```python
from build123d import *

# Parameters (mm, degrees)
SKETCH_1_W          = 44
SKETCH_1_H          = 30
EXTRUDE_1_DEPTH     = 24
SKETCH_5_W          = 20
SKETCH_5_H          = 34.070761632
CUT_EXTRUDE_3_DEPTH = 20
SKETCH_6_R          = 1.5
CUT_EXTRUDE_4_DEPTH = 44
FILLET_1_R          = 2
FILLET_2_R          = 2


# Some blends are built 0.0001 mm under size
with BuildPart() as part:
    # 草图1 → 凸台-拉伸1 (new body)
    with BuildSketch(Plane.XY):
        Rectangle(SKETCH_1_W, SKETCH_1_H)
    extrude(amount=EXTRUDE_1_DEPTH)

    # 草图5 → 切除-拉伸3 (cut)
    with BuildSketch(Plane.XY.offset(24)):
        with Locations((0, 0.619885825)):
            Rectangle(SKETCH_5_W, SKETCH_5_H)
    extrude(amount=-CUT_EXTRUDE_3_DEPTH, mode=Mode.SUBTRACT)

    # 草图6 → 切除-拉伸4 (cut)
    with BuildSketch(Plane(origin=(22, 0, 0), x_dir=(0, 0, -1), z_dir=(1, 0, 0))):
        with Locations((-19, 5)):
            Circle(SKETCH_6_R)
        with Locations((-19, -5)):
            Circle(SKETCH_6_R)
        with Locations((-9, -5)):
            Circle(SKETCH_6_R)
        with Locations((-9, 5)):
            Circle(SKETCH_6_R)
    extrude(amount=-CUT_EXTRUDE_4_DEPTH, mode=Mode.SUBTRACT)

    # 圆角1
    fillet_1_edges = [part.edges().sort_by_distance(p)[0] for p in [
        (-16, -15, 24),
        (-16, 15, 24),
        (16, -15, 24),
        (0, -15, 4),
        (0, 15, 4),
        (-10, 15, 14),
        (-10, -15, 14),
        (10, 15, 14),
        (10, -15, 14),
        (0, -15, 0),
        (0, 15, 0),
        (16, 15, 24),
        (22, -15, 12),
        (-22, -15, 12),
        (-22, 15, 12),
        (22, 15, 12),
    ]]
    fillet(fillet_1_edges, radius=FILLET_1_R - 0.0001)  # a hair under: the kernel refuses the full size

    # 圆角2
    # the kernel refuses this fillet: 2 mm, written as the material it takes off along each edge
    with BuildSketch(Plane(origin=(-12, -15, 22), x_dir=(1, 0, 0), z_dir=(0, 0, -1))) as fillet_2_piece_1:
        with BuildLine():
            CenterArc((0.0001, -1.9999), 1.9999, 0, 90)
            Line((2, -1.9999), (2, 0))
            Line((2, 0), (0.0001, 0))
        make_face()
    revolve(axis=Axis((-12, -15, 22), (0, -1, 0)), revolution_arc=90, mode=Mode.SUBTRACT)
    with BuildSketch(Plane(origin=(-20, -15, 22), x_dir=(0, 0, 1), z_dir=(1, 0, 0))) as fillet_2_piece_2:
        with BuildLine():
            CenterArc((0.0001, -1.9999), 1.9999, 0, 90)
            Line((2, -1.9999), (2, 0))
            Line((2, 0), (0.0001, 0))
        make_face()
    revolve(axis=Axis((-20, -15, 22), (0, -1, 0)), revolution_arc=90, mode=Mode.SUBTRACT)
    with BuildSketch(Plane(origin=(-20, -15, 2), x_dir=(-1, 0, 0), z_dir=(0, 0, 1))) as fillet_2_piece_3:
        with BuildLine():
            CenterArc((0.0001, -1.9999), 1.9999, 0, 90)
            Line((2, -1.9999), (2, 0))
            Line((2, 0), (0.0001, 0))
        make_face()
    revolve(axis=Axis((-20, -15, 2), (0, -1, 0)), revolution_arc=90, mode=Mode.SUBTRACT)
    with BuildSketch(Plane(origin=(20, -15, 2), x_dir=(0, 0, -1), z_dir=(-1, 0, 0))) as fillet_2_piece_4:
        with BuildLine():
            CenterArc((0.0001, -1.9999), 1.9999, 0, 90)
            Line((2, -1.9999), (2, 0))
            Line((2, 0), (0.0001, 0))
        make_face()
    revolve(axis=Axis((20, -15, 2), (0, -1, 0)), revolution_arc=90, mode=Mode.SUBTRACT)
    with BuildSketch(Plane(origin=(12, -15, 22), x_dir=(0, 0, 1), z_dir=(1, 0, 0))) as fillet_2_piece_5:
        with BuildLine():
            CenterArc((0.0001, -1.9999), 1.9999, 0, 90)
            Line((2, -1.9999), (2, 0))
            Line((2, 0), (0.0001, 0))
        make_face()
    revolve(axis=Axis((12, -15, 22), (0, -1, 0)), revolution_arc=90, mode=Mode.SUBTRACT)
    with BuildSketch(Plane(origin=(20, -15, 22), x_dir=(1, 0, 0), z_dir=(0, 0, -1))) as fillet_2_piece_6:
        with BuildLine():
            CenterArc((0.0001, -1.9999), 1.9999, 0, 90)
            Line((2, -1.9999), (2, 0))
            Line((2, 0), (0.0001, 0))
        make_face()
    revolve(axis=Axis((20, -15, 22), (0, -1, 0)), revolution_arc=90, mode=Mode.SUBTRACT)
    with BuildSketch(Plane(origin=(12, 15, 22), x_dir=(-1, 0, 0), z_dir=(0, 0, -1))) as fillet_2_piece_7:
        with BuildLine():
            CenterArc((0.0001, -1.9999), 1.9999, 0, 90)
            Line((2, -1.9999), (2, 0))
            Line((2, 0), (0.0001, 0))
        make_face()
    revolve(axis=Axis((12, 15, 22), (0, 1, 0)), revolution_arc=90, mode=Mode.SUBTRACT)
    with BuildSketch(Plane(origin=(20, 15, 22), x_dir=(0, 0, 1), z_dir=(-1, 0, 0))) as fillet_2_piece_8:
        with BuildLine():
            CenterArc((0.0001, -1.9999), 1.9999, 0, 90)
            Line((2, -1.9999), (2, 0))
            Line((2, 0), (0.0001, 0))
        make_face()
    revolve(axis=Axis((20, 15, 22), (0, 1, 0)), revolution_arc=90, mode=Mode.SUBTRACT)
    with BuildSketch(Plane(origin=(-12, 15, 22), x_dir=(0, 0, 1), z_dir=(-1, 0, 0))) as fillet_2_piece_9:
        with BuildLine():
            CenterArc((0.0001, -1.9999), 1.9999, 0, 90)
            Line((2, -1.9999), (2, 0))
            Line((2, 0), (0.0001, 0))
        make_face()
    revolve(axis=Axis((-12, 15, 22), (0, 1, 0)), revolution_arc=90, mode=Mode.SUBTRACT)
    with BuildSketch(Plane(origin=(20, 15, 2), x_dir=(1, 0, 0), z_dir=(0, 0, 1))) as fillet_2_piece_10:
        with BuildLine():
            CenterArc((0.0001, -1.9999), 1.9999, 0, 90)
            Line((2, -1.9999), (2, 0))
            Line((2, 0), (0.0001, 0))
        make_face()
    revolve(axis=Axis((20, 15, 2), (0, 1, 0)), revolution_arc=90, mode=Mode.SUBTRACT)
    with BuildSketch(Plane(origin=(-20, 15, 22), x_dir=(-1, 0, 0), z_dir=(0, 0, -1))) as fillet_2_piece_11:
        with BuildLine():
            CenterArc((0.0001, -1.9999), 1.9999, 0, 90)
            Line((2, -1.9999), (2, 0))
            Line((2, 0), (0.0001, 0))
        make_face()
    revolve(axis=Axis((-20, 15, 22), (0, 1, 0)), revolution_arc=90, mode=Mode.SUBTRACT)
    with BuildSketch(Plane(origin=(-20, 15, 2), x_dir=(0, 0, -1), z_dir=(1, 0, 0))) as fillet_2_piece_12:
        with BuildLine():
            CenterArc((0.0001, -1.9999), 1.9999, 0, 90)
            Line((2, -1.9999), (2, 0))
            Line((2, 0), (0.0001, 0))
        make_face()
    revolve(axis=Axis((-20, 15, 2), (0, 1, 0)), revolution_arc=90, mode=Mode.SUBTRACT)
    with BuildSketch(Plane(origin=(-22, 15, 0), x_dir=(0, 0, 1), z_dir=(0, -1, 0)), Plane(origin=(-22, 15, 24), x_dir=(1, 0, 0), z_dir=(0, -1, 0)), Plane(origin=(10, -15, 24), x_dir=(0, 0, -1), z_dir=(0, 1, 0))) as fillet_2_piece_13:
        with BuildLine():
            CenterArc((FILLET_2_R, -FILLET_2_R), FILLET_2_R, 90, 90)
            Line((0, -FILLET_2_R), (0, 0))
            Line((0, 0), (FILLET_2_R, 0))
        make_face()
    extrude(amount=30, mode=Mode.SUBTRACT)
    with BuildSketch(Plane(origin=(22, -15, 0), x_dir=(-1, 0, 0), z_dir=(0, 1, 0)), Plane(origin=(22, -15, 24), x_dir=(0, 0, -1), z_dir=(0, 1, 0)), Plane(origin=(-10, 15, 24), x_dir=(-1, 0, 0), z_dir=(0, -1, 0))) as fillet_2_piece_14:
        with BuildLine():
            CenterArc((FILLET_2_R, FILLET_2_R), FILLET_2_R, 180, 90)
            Line((0, FILLET_2_R), (0, 0))
            Line((0, 0), (FILLET_2_R, 0))
        make_face()
    extrude(amount=30, mode=Mode.SUBTRACT)


solid = part.part
```
Can you work these out from the model? Positions are in its coordinate system, mm. A direction names the side the tool comes from. Give positions to 0.01 mm unless a question says otherwise; leave off trailing zeros. Order: outer loops, then holes, each group sorted by start corner. A loop starts at its lowest first (then second) coordinate and runs counter-clockwise, first axis right, second up. Notation, with made-up numbers: M 29,9 L 70,9 A22 ccw 70,47 Z; hole C 57.25,89.5 d8. An arc over 180 degrees is marked long. One line per item, written item: value.
1) On a 3-axis mill with a long thin cutter (end or side, diameter ignored), from which of +Z, -Z, +X, -X, +Y, -Y can I reach the whole of each face in a straight line? I mean faces 5 (the face through (-10.6, -14.43, 11.86)), 6 (the face through (21.4, -0.18, 23.43)), 7 (the face through (0, 0, 4)). Say none if no direction works.
Answer sheet:
face 5: +Z, -Y
face 6: +Z, +X, +Y, -Y
face 7: +Z, +Y, -Y
2) I want a section at D-D, the plane z = 12.75. List the corners of the cut face in (x, y) for me, plus the area to 3 significant figures.
Answer sheet:
outline: M -22,-13 A2 ccw -20,-15 L -12,-15 A2 ccw -10,-13 L -10,13 A2 ccw -12,15 L -20,15 A2 ccw -22,13 Z; M 10,-13 A2 ccw 12,-15 L 20,-15 A2 ccw 22,-13 L 22,13 A2 ccw 20,15 L 12,15 A2 ccw 10,13 Z
area: 713 mm^2
3) I want a section at B-B, the plane y = -5. Count the separate pieces of the cut face and the enclosed holes in it, plus the area to 3 significant figures.
Answer sheet:
separate pieces: 5
enclosed holes: 0
area: 507 mm^2
4) We'd pull the mould along Z, two halves only. Please class faces 1 (the face through (16.08, -4.93, 20.5)), 2 (the face through (16.08, 5.07, 20.5)), 3 (the face through (16, 0, 24)), 4 (the face through (-10.6, 14.43, 11.86)): released by +Z, released by -Z, zero draft, split by the parting line, or undercut.
Answer sheet:
face 1: undercut
face 2: undercut
face 3: released by +Z
face 4: zero draft
5) For P1, Ø6, axis at x = -6, y = 5, coming from the +Z side; P2, Ø1.5, axis at x = -10.5, z = 13.5, coming from the +Y side; P3, Ø3.5, axis at y = 5, z = 9, coming from the +X side, each with a flat end and sliding along its axis, tell me the tip position at first contact or that it passes through.
Answer sheet:
P1: stops at z = 4
P2: stops at y = 14.85
P3: stops at x = 22
6) I want a section at A-A, the plane x = -18. List the corners of the cut face in (y, z) for me.
Answer sheet:
outline: M -15,2 A2 ccw -13,0 L 13,0 A2 ccw 15,2 L 15,22 A2 ccw 13,24 L -13,24 A2 ccw -15,22 Z; hole C -5,9 d3; hole C -5,19 d3; hole C 5,9 d3; hole C 5,19 d3
7) Please list where these lines run through material, in increasing order: line 1 along Y through (x, z) = (-16.25, 9); line 2 along X through (y, z) = (9.5, 7); line 3 along Y through (x, z) = (-17, 8).
Answer sheet:
line 1: y = -15 to -6.5, -3.5 to 3.5, 6.5 to 15
line 2: x = -22 to -10, 10 to 22
line 3: y = -15 to -6.12, -3.88 to 3.88, 6.12 to 15
